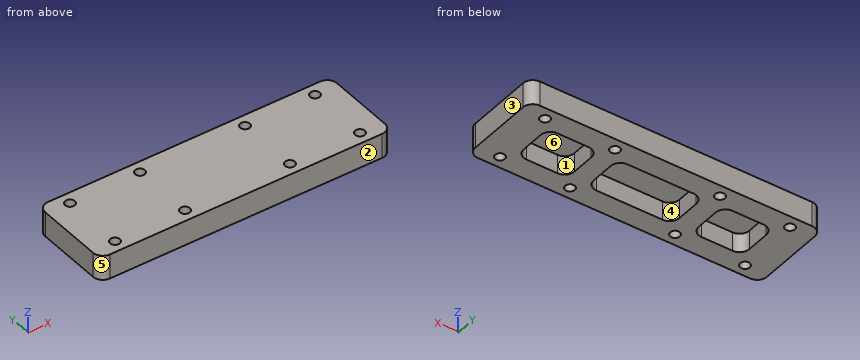
```python
from build123d import *

# Parameters (mm, degrees)
SKETCH1_W           = 150
SKETCH1_H           = 44
SKETCH1_R           = 2.5
BOSS_EXTRUDE1_DEPTH = 12.7
FILLET1_R           = 5
SKETCH7_W           = 26
SKETCH7_H           = 22
SKETCH7_W_2         = 44
CUT_EXTRUDE2_DEPTH  = 9.7
FILLET3_R           = 5


with BuildPart() as part:
    # Sketch1 → Boss-Extrude1 (new body)
    with BuildSketch(Plane.XY):
        Rectangle(SKETCH1_W, SKETCH1_H)
        with Locations((-63, -16)):
            Circle(SKETCH1_R, mode=Mode.SUBTRACT)
        with Locations((-63, 16)):
            Circle(SKETCH1_R, mode=Mode.SUBTRACT)
        with Locations((-27, -16)):
            Circle(SKETCH1_R, mode=Mode.SUBTRACT)
        with Locations((-27, 16)):
            Circle(SKETCH1_R, mode=Mode.SUBTRACT)
        with Locations((27, -16)):
            Circle(SKETCH1_R, mode=Mode.SUBTRACT)
        with Locations((27, 16)):
            Circle(SKETCH1_R, mode=Mode.SUBTRACT)
        with Locations((63, -16)):
            Circle(SKETCH1_R, mode=Mode.SUBTRACT)
        with Locations((63, 16)):
            Circle(SKETCH1_R, mode=Mode.SUBTRACT)
    extrude(amount=BOSS_EXTRUDE1_DEPTH)

    # Fillet1
    fillet1_edges = [part.edges().sort_by_distance(p)[0] for p in [
        (75, -22, 6.35),
        (-75, -22, 6.35),
        (-75, 22, 6.35),
        (75, 22, 6.35),
    ]]
    fillet(fillet1_edges, radius=FILLET1_R)

    # Sketch7 → Cut-Extrude2 (cut)
    with BuildSketch(Plane(origin=(0, 0, 0), x_dir=(-1, 0, 0), z_dir=(0, 0, -1))):
        with Locations((-45, 0)):
            Rectangle(SKETCH7_W, SKETCH7_H)
        Rectangle(SKETCH7_W_2, SKETCH7_H)
        with Locations((45, 0)):
            Rectangle(SKETCH7_W, SKETCH7_H)
    extrude(amount=-CUT_EXTRUDE2_DEPTH, mode=Mode.SUBTRACT)

    # Fillet3
    fillet3_edges = [part.edges().sort_by_distance(p)[0] for p in [
        (58, -11, 4.85),
        (58, 11, 4.85),
        (32, 11, 4.85),
        (32, -11, 4.85),
        (22, -11, 4.85),
        (22, 11, 4.85),
        (-22, 11, 4.85),
        (-22, -11, 4.85),
        (-32, -11, 4.85),
        (-32, 11, 4.85),
        (-58, 11, 4.85),
        (-58, -11, 4.85),
    ]]
    fillet(fillet3_edges, radius=FILLET3_R)


solid = part.part
```
Can you work these out from the model? Positions are in its coordinate system, mm. Face numbers are marked on the shaded views. A direction names the side the tool comes from. Give positions to 0.01 mm unless a question says otherwise; leave off trailing zeros. Loops run counter-clockwise (first coordinate to the right, second up) from the corner with the lowest first, then second, coordinate; pieces in that order, holes last. Notation, with made-up numbers: M 10,-31 L 21,-31 A25 ccw 21,-2 Z; hole C 3.5,21.25 d4. An arc over 180 degrees is marked long. Use one line per item in the form item = value. Start each with the question number.
(1) I'm going to push a flat-ended pin straight in: P1, Ø17.5, axis at x = 3, y = 1.5, coming from the -Z side. Where does the tip first touch, or does it pass through?
(2) On a 3-axis mill with a long thin cutter (end or side, diameter ignored), from which of +Z, -Z, +X, -X, +Y, -Y can I reach the whole of each face in a straight line? I mean the marked faces 5 and 6. Say none if no direction works.
(3) Please list where these lines run through material, in increasing order: line 1 (Y direction, x = -27, z = 3.75); line 2 (X direction, y = -1, z = 6.5); line 3 (Y direction, x = -6, z = 3.5).
(4) I want a section at C-C, the plane x = -34.5. Write out the boundary of the cut face in (y, z).
(5) Thinking about a two-plate mould opening in X: for the marked faces 1, 2, 3 and 4, which applies, released by +X, released by -X, zero draft, split by the parting line, or undercut?
(6) I want a section at A-A, the plane x = 27. Write out the boundary of the cut face in (y, z), and give its area (3 significant figures).
(7) I want a section at D-D, the plane y = -8. Write out the boundary of the cut face in (x, z), and give its area (3 significant figures).
(8) I want a section at B-B, the plane z = 3.75. State how many separate pieces and enclosed holes the cut face has, and give its area (3 significant figures).
Worked out:
q1.P1 = 9.7
q2.face_5 = +Z, -Z, -X, -Y
q2.face_6 = -Z
q3.line_1 = -22 to -18.5, -13.5 to 13.5, 18.5 to 22
q3.line_2 = -75 to -58, -32 to -22, 22 to 32, 58 to 75
q3.line_3 = -22 to -11, 11 to 22
q4.outline = M -22,0 L -10.33,0 L -10.33,9.7 L 10.33,9.7 L 10.33,0 L 22,0 L 22,12.7 L -22,12.7 Z
q5.face_1 = undercut
q5.face_2 = zero draft
q5.face_3 = released by +X
q5.face_4 = undercut
q6.outline = M -22,0 L -18.5,0 L -18.5,12.7 L -22,12.7 Z; M -13.5,0 L 13.5,0 L 13.5,12.7 L -13.5,12.7 Z; M 18.5,0 L 22,0 L 22,12.7 L 18.5,12.7 Z
q6.area = 432 mm²
q7.outline = M -75,0 L -57.58,0 L -57.58,9.7 L -32.42,9.7 L -32.42,0 L -21.58,0 L -21.58,9.7 L 21.58,9.7 L 21.58,0 L 32.42,0 L 32.42,9.7 L 57.58,9.7 L 57.58,0 L 75,0 L 75,12.7 L -75,12.7 Z
q7.area = 998 mm²
q8.separate_pieces = 1
q8.enclosed_holes = 11
q8.area = 4,370 mm²
